Here's how the part is built. I have some questions about the finished solid (model axes, mm). Face numbers are marked on the shaded views. Round coordinates to 2 decimals unless told otherwise and drop trailing zeros. Write each loop counter-clockwise with the first axis right and the second up, starting at its lowest first coordinate (ties: lowest second). Pieces come first, ordered by that corner, then holes. Notation, with made-up numbers: (-25.75, 43) -> (1.25, 43) arc R10 ccw to (1.25, 49) -> close; hole circle Ø8 at (-28, -17.75). An arc over 180 degrees is marked (long way). Answer as CSV lines item,"result".
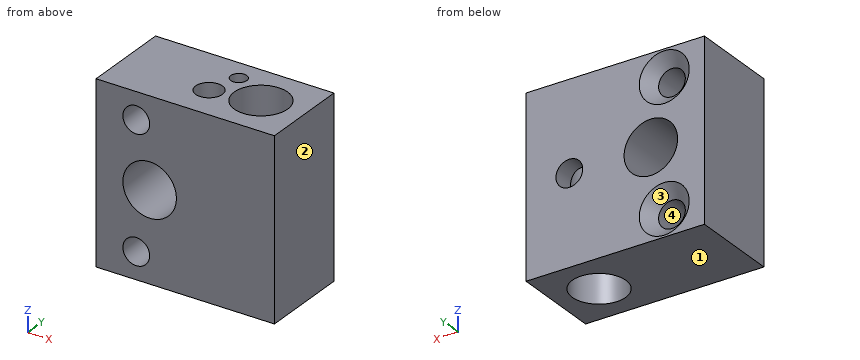
```python
from build123d import *

# Parameters (mm, degrees)
SKETCH1_W                                       = 20
SKETCH1_H                                       = 20
BOSS_EXTRUDE1_DEPTH                             = 10
F_6_0MM_DOWEL_HOLE2_D                           = 6
CSK_FOR_M3_FLAT_HEAD_MACHINE_SCREW1_D           = 3
CSK_FOR_M3_FLAT_HEAD_MACHINE_SCREW1_CSINK_D     = 5.6
CSK_FOR_M3_FLAT_HEAD_MACHINE_SCREW1_CSINK_ANGLE = 90
F_6_0MM_DOWEL_HOLE3_D                           = 6
F_3_0MM_DOWEL_HOLE1_REACH                       = 32
F_3_0MM_DOWEL_HOLE1_BORE_R                      = 1.5
F_3_0MM_DOWEL_HOLE2_D                           = 3
F_3_0MM_DOWEL_HOLE2_DEPTH                       = 6
F_3_0MM_DOWEL_HOLE2_TIP                         = 0.901290929
F_1_5MM_DOWEL_HOLE1_D                           = 1.8
F_1_5MM_DOWEL_HOLE1_DEPTH                       = 4
F_1_5MM_DOWEL_HOLE1_TIP                         = 0.540774557


with BuildPart() as part:
    # Sketch1 → Boss-Extrude1 (new body)
    with BuildSketch(Plane(origin=(0, 0, 0), x_dir=(1, 0, 0), z_dir=(0, 1, 0))):
        with Locations((10, 10)):
            Rectangle(SKETCH1_W, SKETCH1_H)
    extrude(amount=BOSS_EXTRUDE1_DEPTH)

    # Ø6.0mm Dowel Hole2 (through all)
    with Locations(Plane(origin=(0, 10, 0), x_dir=(1, 0, 0), z_dir=(0, 1, 0))):
        with Locations((6.01, 10)):
            Hole(F_6_0MM_DOWEL_HOLE2_D / 2)

    # CSK for M3 Flat Head Machine Screw1 (through all)
    with Locations(Plane(origin=(0, 10, 0), x_dir=(1, 0, 0), z_dir=(0, 1, 0))):
        with Locations((4.51, 3), (4.51, 17)):
            CounterSinkHole(CSK_FOR_M3_FLAT_HEAD_MACHINE_SCREW1_D / 2, CSK_FOR_M3_FLAT_HEAD_MACHINE_SCREW1_CSINK_D / 2, counter_sink_angle=CSK_FOR_M3_FLAT_HEAD_MACHINE_SCREW1_CSINK_ANGLE)

    # Ø6.0mm Dowel Hole3 (through all)
    with Locations(Plane.XY):
        with Locations((15.15, 5)):
            Hole(F_6_0MM_DOWEL_HOLE3_D / 2)

    # Ø3.0mm Dowel Hole1 bore → Ø3.0mm Dowel Hole1 (cut, up to next)
    with BuildSketch(Plane(origin=(0, 10, 0), x_dir=(1, 0, 0), z_dir=(0, 1, 0)), mode=Mode.PRIVATE) as f_3_0mm_dowel_hole1_sk1:
        with Locations((15.15, 10)):
            Circle(F_3_0MM_DOWEL_HOLE1_BORE_R)
    f_3_0mm_dowel_hole1_tool1 = extrude(f_3_0mm_dowel_hole1_sk1.sketch, amount=-F_3_0MM_DOWEL_HOLE1_REACH, mode=Mode.PRIVATE) & part.part
    add(f_3_0mm_dowel_hole1_tool1.solids().sort_by_distance((15.15, 10, -10))[0], mode=Mode.SUBTRACT)

    # Ø3.0mm Dowel Hole2
    with Locations(Plane.XY):
        with Locations((10, 4)):
            Hole(F_3_0MM_DOWEL_HOLE2_D / 2, depth=F_3_0MM_DOWEL_HOLE2_DEPTH)
            with Locations((0, 0, -(F_3_0MM_DOWEL_HOLE2_DEPTH + F_3_0MM_DOWEL_HOLE2_TIP / 2))):  # 118° drill point
                Cone(0, F_3_0MM_DOWEL_HOLE2_D / 2, F_3_0MM_DOWEL_HOLE2_TIP, mode=Mode.SUBTRACT)

    # Ø1.5mm Dowel Hole1
    with Locations(Plane.XY):
        with Locations((11, 7.5)):
            Hole(F_1_5MM_DOWEL_HOLE1_D / 2, depth=F_1_5MM_DOWEL_HOLE1_DEPTH)
            with Locations((0, 0, -(F_1_5MM_DOWEL_HOLE1_DEPTH + F_1_5MM_DOWEL_HOLE1_TIP / 2))):  # 118° drill point
                Cone(0, F_1_5MM_DOWEL_HOLE1_D / 2, F_1_5MM_DOWEL_HOLE1_TIP, mode=Mode.SUBTRACT)


solid = part.part
```
1. If I drill on line 1 (X direction, y = 4.5, z = -9.5); line 2 (X direction, y = 3.75, z = -10); line 3 (Y direction, x = 10, z = -4.2), over which ranges is the centre line in solid material (lowest first)?
Numbers:
line 1,"x = 0 to 3.05, 8.97 to 12.19, 18.11 to 20"
line 2,"x = 0 to 3.01, 9.01 to 12.42, 17.88 to 20"
line 3,"y = 0 to 2.5, 5.5 to 10"
2. Suppose I cut it at B-B on z = -17. Please give me the cut outline in (x, y), and give its area (3 significant figures).
Numbers:
outline,"(0, 0) -> (3.01, 0) -> (3.01, 8.7) -> (1.71, 10) -> (0, 10) -> close; (6.01, 0) -> (20, 0) -> (20, 10) -> (7.31, 10) -> (6.01, 8.7) -> close; hole circle Ø6 at (15.15, 5)"
area,"140 mm^2"
3. Suppose I cut it at C-C on x = 17.5. Please give me the cut outline in (y, z).
Numbers:
outline,"(0, -20) -> (3.14, -20) -> (3.14, 0) -> (0, 0) -> close; (6.86, -20) -> (10, -20) -> (10, 0) -> (6.86, 0) -> close"
4. Suppose I cut it at D-D on x = 15.5. Please give me the cut outline in (y, z).
Numbers:
outline,"(0, -20) -> (2.02, -20) -> (2.02, 0) -> (0, 0) -> close; (7.98, -20) -> (10, -20) -> (10, -11.46) -> (7.98, -11.46) -> close; (7.98, -8.54) -> (10, -8.54) -> (10, 0) -> (7.98, 0) -> close"
5. If we mould it in two halves opening along X, with no side actions, what happens to the marked faces 1, 2, 3 and 4? For each: released by +X, released by -X, zero draft, split by the parting line, or undercut.
Numbers:
face 1,"zero draft"
face 2,"released by +X"
face 3,"undercut"
face 4,"undercut"
6. Suppose I cut it at A-A on z = -3. Please give me the cut outline in (x, y).
Numbers:
outline,"(0, 0) -> (3.01, 0) -> (3.01, 8.7) -> (1.71, 10) -> (0, 10) -> close; (6.01, 0) -> (20, 0) -> (20, 10) -> (7.31, 10) -> (6.01, 8.7) -> close; hole circle Ø3 at (10, 4); hole circle Ø1.8 at (11, 7.5); hole circle Ø6 at (15.15, 5)"
7. For pin 1 Ø4 at (x, z) = (4.51, -17) entering from +Y; pin 2 Ø2.5 at (x, y) = (10, 4) entering from +Z, each with a flat end and sliding along its axis, tell me the tip position at first contact or that it passes through.
Numbers:
pin 1,"stops at y = 9.2"
pin 2,"stops at z = -6.15"
